```python
from build123d import *

# Parameters (mm, degrees)
SKETCH_1_W      = 66.6
SKETCH_1_H      = 8
SKETCH_1_R      = 1.6
EXTRUDE_1_DEPTH = 5
SKETCH_2_W      = 8
SKETCH_2_H      = 20
EXTRUDE_2_DEPTH = 8
FILLET_1_R      = 2
FILLET_2_R      = 5
FILLET_3_R      = 2


with BuildPart() as part:
    # 草图1 → 凸台-拉伸1 (new body)
    with BuildSketch(Plane.XY):
        Rectangle(SKETCH_1_W, SKETCH_1_H)
        with Locations((-29.3, 0)):
            Circle(SKETCH_1_R, mode=Mode.SUBTRACT)
        with Locations(Location((29.3, 0, 0), (0, 0, 180))):
            Circle(SKETCH_1_R, mode=Mode.SUBTRACT)
    extrude(amount=EXTRUDE_1_DEPTH)

    # 草图2 → 凸台-拉伸2 (add)
    with BuildSketch(Plane(origin=(0, 4, 0), x_dir=(1, 0, 0), z_dir=(0, 1, 0))):
        with Locations((0, 10)):
            Rectangle(SKETCH_2_W, SKETCH_2_H)
    extrude(amount=-EXTRUDE_2_DEPTH)

    # 圆角1
    fillet_1_edges = [part.edges().sort_by_distance(p)[0] for p in [
        (-33.3, 4, 2.5),
        (33.3, 4, 2.5),
        (33.3, -4, 2.5),
        (-33.3, -4, 2.5),
    ]]
    fillet(fillet_1_edges, radius=FILLET_1_R)

    # 圆角2
    fillet_2_edges = [part.edges().sort_by_distance(p)[0] for p in [
        (4, 0, 0),
        (-4, 0, 0),
    ]]
    fillet(fillet_2_edges, radius=FILLET_2_R)

    # 圆角3
    fillet_3_edges = [part.edges().sort_by_distance(p)[0] for p in [
        (-4, 0, -20),
        (4, 0, -20),
    ]]
    fillet(fillet_3_edges, radius=FILLET_3_R)


solid = part.part
```
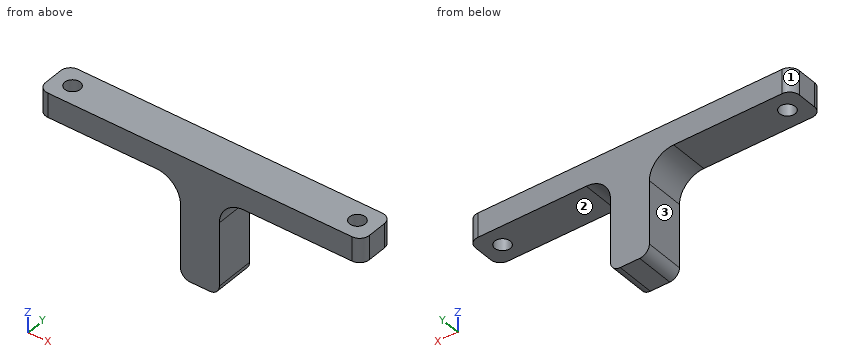
Input: part model. Units: mm. Frame: model coordinates. Face numbers are marked on the shaded views. A direction names the side the tool comes from. Give positions to 0.01 mm unless a question says otherwise; leave off trailing zeros. Write each loop counter-clockwise with the first axis right and the second up, starting at its lowest first coordinate (ties: lowest second). Pieces come first, ordered by that corner, then holes. Notation, with made-up numbers: (62.5, 50) - (93.5, 50) arc R19 ccw to (93.5, 59) - close; hole circle Ø10 at (56, -5). An arc over 180 degrees is marked (long way). Write item = value, one per line. Start each with the question number.
1. Section query B-B, the plane x = -29.3. Output: boundary loops of the cut face in (y, z), then the cut area to 3 significant figures.
2. Access query for the marked faces 1, 2 and 3. Directions: +Z, -Z, +X, -X, +Y, -Y. A direction counts if a zero-diameter tool reaches every point of the face in a straight line with its end or side. Return the directions, or none.
3. Section query D-D, the plane x = 26. Output: boundary loops of the cut face in (y, z), then the cut area to 3 significant figures.
4. First-contact query: pin 1 Ø2 at (y, z) = (-3, 2) entering from +X; pin 2 Ø2.5 at (x, y) = (-29.3, 0) entering from +Z; pin 3 Ø4 at (y, z) = (0.5, -12) entering from +X; pin 4 Ø4 at (x, y) = (-24.5, -0.5) entering from -Z. Flat tips, straight axial feed; report the tip coordinate or a pass-through.
5. Section query C-C, the plane z = -9. Output: boundary loops of the cut face in (x, y), then the cut area to 3 significant figures.
6. Section query A-A, the plane y = 0. Output: boundary loops of the cut face in (x, z), then the cut area to 3 significant figures.
7. Ray query, L1, parallel to Y at x = -29.3, z = 3.65; L2, parallel to X at y = -3.5, z = -9.25; L3, parallel to Z at x = 5, y = -0.5. Return the intervals inside material, ascending.
Check sheet entries:
q1.outline = (-4, 0) - (-1.6, 0) - (-1.6, 5) - (-4, 5) - close; (1.6, 0) - (4, 0) - (4, 5) - (1.6, 5) - close
q1.area = 24.0 mm2
q2.face_1 = +Z, -Z, -X, +Y
q2.face_2 = -Z, +X, +Y, -Y
q2.face_3 = -Z, -X, +Y, -Y
q3.outline = (-4, 0) - (4, 0) - (4, 5) - (-4, 5) - close
q3.area = 40.0 mm2
q4.pin_1 = 33.3
q4.pin_2 = through
q4.pin_3 = 4
q4.pin_4 = 0
q5.outline = (-4, -4) - (4, -4) - (4, 4) - (-4, 4) - close
q5.area = 64.0 mm2
q6.outline = (-33.3, 0) - (-30.9, 0) - (-30.9, 5) - (-33.3, 5) - close; (-27.7, 0) - (-9, 0) arc R5 cw to (-4, -5) - (-4, -18) arc R2 ccw to (-2, -20) - (2, -20) arc R2 ccw to (4, -18) - (4, -5) arc R5 cw to (9, 0) - (27.7, 0) - (27.7, 5) - (-27.7, 5) - close; (30.9, 0) - (33.3, 0) - (33.3, 5) - (30.9, 5) - close
q6.area = 470 mm2
q7.L1 = -4 to -1.6, 1.6 to 4
q7.L2 = -4 to 4
q7.L3 = -2 to 5
